from build123d import *

# Parameters (mm, degrees)
HEX_2_DEPTH                 = 10
M3X1_0_FEMALE_THREADS_D     = 2.5
M3X1_0_FEMALE_THREADS_DEPTH = 7.5
M3X1_0_FEMALE_THREADS_TIP   = 0.751075774
M3X1_0_START                = 5
SKETCH2_R                   = 1.25
M3X1_0_MALE_THREADS_DEPTH   = 5


with BuildPart() as part:
    # Sketch1 → Hex 2 (new body)
    with BuildSketch(Plane(origin=(0, 0, 0), x_dir=(1, 0, 0), z_dir=(0, 1, 0))):
        Polygon((2.886751346, 0), (1.443375673, 2.5), (-1.443375673, 2.5), (-2.886751346, 0), (-1.443375673, -2.5), (1.443375673, -2.5), align=None)
    extrude(amount=HEX_2_DEPTH)

    # M3x1.0 Female Threads
    with Locations(Plane.XZ):
        with Locations((0, 0)):
            Hole(M3X1_0_FEMALE_THREADS_D / 2, depth=M3X1_0_FEMALE_THREADS_DEPTH)
            with Locations((0, 0, -(M3X1_0_FEMALE_THREADS_DEPTH + M3X1_0_FEMALE_THREADS_TIP / 2))):  # 118° drill point
                Cone(0, M3X1_0_FEMALE_THREADS_D / 2, M3X1_0_FEMALE_THREADS_TIP, mode=Mode.SUBTRACT)

    # Sketch2 → M3x1.0 Male Threads (add)
    with BuildSketch(Plane(origin=(0, 10, 0), x_dir=(-1, 0, 0), z_dir=(0, 1, 0)).offset(M3X1_0_START)):
        with Locations(Location((0, 0, 0), (0, 0, 270))):
            Circle(SKETCH2_R)
    extrude(amount=-M3X1_0_MALE_THREADS_DEPTH)


solid = part.part
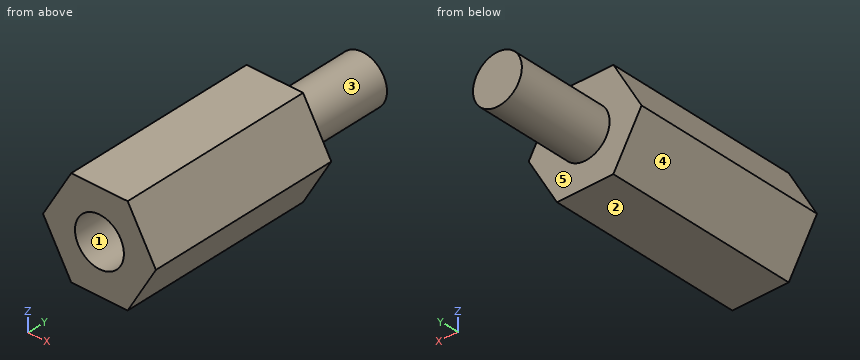
Input: part model. Units: mm. Frame: model coordinates. Face numbers are marked on the shaded views. A direction names the side the tool comes from. Coordinates: 2 decimals unless noted, no trailing zeros. Loops run counter-clockwise (first coordinate to the right, second up) from the corner with the lowest first, then second, coordinate; pieces in that order, holes last.
(1) Section A-A on y = 5. Return the cut outline in (x, z), then the cut area to 3 significant figures.
(2) Section D-D on x = 1.8. Return the cut outline in (y, z).
(3) Pull-direction query (Z, two-part tool) for the marked faces 1, 2 and 3; classes: released by +Z, released by -Z, zero draft, split by the parting line, or undercut.
(4) Section B-B on x = -1.75. Return the cut outline in (y, z), then the cut area to 3 significant figures.
(5) Material intervals for probe 1 along Z at (x, y) = (0, 1.5); probe 2 along Y at (x, z) = (-1.95, -1.3); probe 3 along Z at (x, y) = (-0.1, 10.5), sorted ascending.
(6) Section C-C on y = 13.5. Return the cut outline in (x, z), then the cut area to 3 significant figures.
(7) Set-up query: the marked faces 4 and 5. Return all of +Z, -Z, +X, -X, +Y, -Y with unobstructed straight access to the full face (end or side cutting, diameter ignored); none if empty.
Data:
1. outline: (-2.89, 0) - (-1.44, -2.5) - (1.44, -2.5) - (2.89, 0) - (1.44, 2.5) - (-1.44, 2.5) - close; hole circle Ø2.5 at (0, 0)
1. area: 16.7 mm2
2. outline: (0, -1.88) - (10, -1.88) - (10, 1.88) - (0, 1.88) - close
3. face 1: undercut
3. face 2: released by -Z
3. face 3: split by the parting line
4. outline: (0, -1.97) - (10, -1.97) - (10, 1.97) - (0, 1.97) - close
4. area: 39.4 mm2
5. probe 1: z = -2.5 to -1.25, 1.25 to 2.5
5. probe 2: y = 0 to 10
5. probe 3: z = -1.25 to 1.25
6. outline: circle Ø2.5 at (0, 0)
6. area: 4.91 mm2
7. face 4: -Z, -X, +Y, -Y
7. face 5: +Y
